from build123d import *

# Parameters (mm, degrees)
F0_W     = 12.7
F0_H     = 47.625
F1_DEPTH = 3.175
F2_W     = 30
F2_H     = 70
F3_DEPTH = 2.54
F5_D     = 3.4544
F5_DEPTH = 15.08125
F5_TIP   = 1.0378064612
F7_D     = 2.7051
F7_DEPTH = 15.0876
F7_TIP   = 0.8126940303


with BuildPart() as f1:
    # F0 (on Top) → F1 (new body)
    with BuildSketch(Plane.XY):
        Rectangle(F0_W, F0_H)
    extrude(amount=F1_DEPTH)

    # F2 (on face) → F3 (join)
    with BuildSketch(Plane.XY.offset(3.175)):
        Rectangle(F2_W, F2_H)
    extrude(amount=F3_DEPTH)

    # F5
    with Locations(Plane(origin=(0, 0, 0), x_dir=(1, 0, 0), z_dir=(0, 0, -1))):
        with Locations((0, 15.875), (0, 0), (0, -15.875)):
            Hole(F5_D / 2, depth=F5_DEPTH)
            with Locations((0, 0, -(F5_DEPTH + F5_TIP / 2))):  # 118° drill point
                Cone(0, F5_D / 2, F5_TIP, mode=Mode.SUBTRACT)

    # F7
    with Locations(Plane(origin=(0, 0, 3.175), x_dir=(1, 0, 0), z_dir=(0, 0, -1))):
        with Locations((0, 28.575), (0, -28.575)):
            Hole(F7_D / 2, depth=F7_DEPTH)
            with Locations((0, 0, -(F7_DEPTH + F7_TIP / 2))):  # 118° drill point
                Cone(0, F7_D / 2, F7_TIP, mode=Mode.SUBTRACT)


solid = f1.part
Verification items for the finished model (mm, model axes). A direction names the side the tool comes from. Coordinates: 2 decimals unless noted, no trailing zeros. Order: outer loops, then holes, each group sorted by start corner. A loop starts at its lowest first (then second) coordinate and runs counter-clockwise, first axis right, second up. Notation, with made-up numbers: (27, 32.5) -> (73, 32.5) arc R26 ccw to (73, 62.5) -> close; hole circle Ø7 at (-4, -11.5). An arc over 180 degrees is marked (long way). Put each result on its own line as item: value. Start each with the question number.
1. Go/stop test with flat-tipped pins: pin 1 Ø1.5 at (y, z) = (-3, 1) entering from +X; pin 2 Ø1.5 at (y, z) = (11.5, 1) entering from -X; pin 3 Ø2.5 at (x, z) = (0.5, 1) entering from -Y. Record where each tip stops, or that it passes through.
2. Cross-section at D-D, the plane x = 3.75. Record the boundary of the cut face in (y, z) (1 decimal), then the cut area to 3 significant figures.
3. Mould release check, pull along X, two halves, no side actions. Record for faces 1 (the cylindrical face through (-0.624, -27.375, 4.463)), 2 (the flat face through (-15, 0, 4)), 3 (the flat face through (3, 0, 0)): released by +X, released by -X, zero draft, split by the parting line, or undercut.
4. Material ranges on L1, parallel to Y at x = 0, z = 2.3; L2, parallel to Y at x = 0, z = 3.35; L3, parallel to Y at x = 0.25, z = 2.1, recorded low to high. Write a range as [from, to].
5. Cross-section at C-C, the plane z = 4.65. Record the boundary of the cut face in (x, y) (3 decimals), then the cut area to 3 significant figures.
6. Cross-section at A-A, the plane y = 0. Record the boundary of the cut face in (x, z) (3 decimals).
7. Cross-section at B-B, the plane x = 0. Record the boundary of the cut face in (y, z) (1 decimal), then the cut area to 3 significant figures.
8. Access from +Z, -Z, +X, -X, +Y, -Y to the whole of each face (thin tool, end or side, straight path). Record for faces 4 (the flat face through (-6.35, 0, 2)), 5 (the flat face through (0, -23.812, 2)), 6 (the flat face through (0, 23.812, 2)).
Computed:
1. pin 1: x = 6.35
1. pin 2: x = -6.35
1. pin 3: y = -23.81
2. outline: (-35, 3.2) -> (-23.8, 3.2) -> (-23.8, 0) -> (23.8, 0) -> (23.8, 3.2) -> (35, 3.2) -> (35, 5.7) -> (-35, 5.7) -> close
2. area: 329 mm2
3. face 1: undercut
3. face 2: released by -X
3. face 3: zero draft
4. L1: [-23.81, -17.6], [-14.15, -1.73], [1.73, 14.15], [17.6, 23.81]
4. L2: [-35, -29.93], [-27.22, -17.6], [-14.15, -1.73], [1.73, 14.15], [17.6, 27.22], [29.93, 35]
4. L3: [-23.81, -17.58], [-14.17, -1.71], [1.71, 14.17], [17.58, 23.81]
5. outline: (-15, -35) -> (15, -35) -> (15, 35) -> (-15, 35) -> close; hole circle Ø3.454 at (0, -15.875); hole circle Ø3.454 at (0, 0); hole circle Ø3.454 at (0, 15.875); hole circle Ø2.705 at (0, -28.575); hole circle Ø2.705 at (0, 28.575)
5. area: 2,060 mm2
6. outline: (-15, 3.175) -> (-6.35, 3.175) -> (-6.35, 0) -> (-1.727, 0) -> (-1.727, 5.715) -> (-15, 5.715) -> close; (1.727, 0) -> (6.35, 0) -> (6.35, 3.175) -> (15, 3.175) -> (15, 5.715) -> (1.727, 5.715) -> close
7. outline: (-35, 3.2) -> (-29.9, 3.2) -> (-29.9, 5.7) -> (-35, 5.7) -> close; (-27.2, 3.2) -> (-23.8, 3.2) -> (-23.8, 0) -> (-17.6, 0) -> (-17.6, 5.7) -> (-27.2, 5.7) -> close; (-14.1, 0) -> (-1.7, 0) -> (-1.7, 5.7) -> (-14.1, 5.7) -> close; (1.7, 0) -> (14.1, 0) -> (14.1, 5.7) -> (1.7, 5.7) -> close; (17.6, 0) -> (23.8, 0) -> (23.8, 3.2) -> (27.2, 3.2) -> (27.2, 5.7) -> (17.6, 5.7) -> close; (29.9, 3.2) -> (35, 3.2) -> (35, 5.7) -> (29.9, 5.7) -> close
7. area: 256 mm2
8. face 4: -Z, -X, +Y, -Y
8. face 5: -Z, +X, -X, -Y
8. face 6: -Z, +X, -X, +Y
